The model under review builds one solid part; all positions refer to its coordinate system, in mm. A direction names the side the tool comes from. Give positions to 0.01 mm unless a question says otherwise; leave off trailing zeros. Loops run counter-clockwise (first coordinate to the right, second up) from the corner with the lowest first, then second, coordinate; pieces in that order, holes last. Notation, with made-up numbers: M -16,-7 L 0,-7 A17 cw 0,22 Z; hole C 35,-26.75 d8. An arc over 180 degrees is marked long. One line per item, written item: value. Start each with the question number.
Q1. We need section C-C on y = 0.7. Give the number of separate pieces and of enclosed holes in the cut face, plus the area to 3 significant figures.
Q2. We need section B-B on x = -39. Write out the cut boundary in (y, z).
Q3. For faces 1 (the face through (46.52, 0.69, 39.04)), 2 (the face through (-46.57, 0.69, 38.98)), 3 (the face through (-44.7, 0.69, -45.04)), 4 (the face through (-38.86, 0.689, 46.664)), 5 (the face through (38.86, 0.689, -46.664)), list the 3-axis set-ups (+Z, -Z, +X, -X, +Y, -Y) from which the entire face can be reached by the end or side of a thin tool; tool diameter is ignored.
Q4. Mouldability with a two-part tool opening along Z and no side actions: class faces 6 (the face through (-39.9, 0.7, -25.7)), 7 (the face through (44.7, 0.69, 45.04)), 8 (the face through (-38.8, 0.69, -46.71)), 9 (the face through (-1, 1.397, -1)) as released by +Z, released by -Z, zero draft, split by the parting line, or undercut.
Q5. We need section A-A on z = 24.5. Write out the cut boundary in (x, y), plus the area to 3 significant figures.
Q6. We need section D-D on z = -38. Write out the cut boundary in (x, y), plus the area to 3 significant figures.
Q7. To check wall thickness, follow line 1 along X through (y, z) = (0.5, -36); line 2 along Z through (x, y) = (-40, 1.3); line 3 along X through (y, z) = (0.5, 35). State the ranges of each line that lie inside material, in increasing order. Write a range as from..to.
```python
from build123d import *

# Parameters (mm, degrees)
SKETCH1_R           = 1.016000002
SKETCH1_R_2         = 1.015999994
SKETCH1_R_3         = 1.016000004
SKETCH1_R_4         = 1.016000003
SKETCH1_R_5         = 1.5
BOSS_EXTRUDE1_DEPTH = 1.397


with BuildPart() as part:
    # Sketch1 → Boss-Extrude1 (new body)
    with BuildSketch(Plane(origin=(0, 0, 0), x_dir=(1, 0, 0), z_dir=(0, 1, 0))):
        with BuildLine():
            Line((-44.657487237, -41.209177315), (-46.396043566, -42.947733643))
            ThreePointArc((-46.396043566, -42.947733643), (-46.47043426, -43.125880979), (-46.398093321, -43.304870469))
            Line((-46.398093321, -43.304870469), (-43.050556902, -46.730153436))
            ThreePointArc((-43.050556902, -46.730153436), (-42.865374913, -46.831022486), (-42.667823962, -46.757262364))
            Line((-42.667823962, -46.757262364), (-40.871772737, -44.96121114))
            ThreePointArc((-40.871772737, -44.96121114), (-38.831009329, -46.687575031), (-36.702263747, -48.304204185))
            ThreePointArc((-36.702263747, -48.304204185), (-35.216668272, -49.053976946), (-33.572746514, -49.312190732))
            Line((-33.572746514, -49.312190732), (33.572746514, -49.312190732))
            ThreePointArc((33.572746514, -49.312190732), (35.216668272, -49.053976946), (36.702263747, -48.304204185))
            ThreePointArc((36.702263747, -48.304204185), (38.831009329, -46.687575031), (40.871772737, -44.96121114))
            Line((40.871772737, -44.96121114), (42.667823962, -46.757262364))
            ThreePointArc((42.667823962, -46.757262364), (42.865374913, -46.831022486), (43.050556902, -46.730153436))
            Line((43.050556902, -46.730153436), (46.398093321, -43.304870469))
            ThreePointArc((46.398093321, -43.304870469), (46.47043426, -43.125880979), (46.396043566, -42.947733643))
            Line((46.396043566, -42.947733643), (44.657487237, -41.209177315))
            ThreePointArc((44.657487237, -41.209177315), (46.545191327, -39.007785053), (48.304204175, -36.702263762))
            ThreePointArc((48.304204175, -36.702263762), (49.053976936, -35.216668286), (49.312190722, -33.572746527))
            Line((49.312190722, -33.572746527), (49.312190722, 33.572746527))
            ThreePointArc((49.312190722, 33.572746527), (49.053976936, 35.216668286), (48.304204175, 36.702263762))
            ThreePointArc((48.304204175, 36.702263762), (46.545191327, 39.007785053), (44.657487237, 41.209177315))
            Line((44.657487237, 41.209177315), (46.396043566, 42.947733643))
            ThreePointArc((46.396043566, 42.947733643), (46.47043426, 43.125880979), (46.398093321, 43.304870469))
            Line((46.398093321, 43.304870469), (43.050556902, 46.730153436))
            ThreePointArc((43.050556902, 46.730153436), (42.865374913, 46.831022486), (42.667823962, 46.757262364))
            Line((42.667823962, 46.757262364), (40.871772737, 44.96121114))
            ThreePointArc((40.871772737, 44.96121114), (38.831009329, 46.687575031), (36.702263747, 48.304204185))
            ThreePointArc((36.702263747, 48.304204185), (35.216668272, 49.053976946), (33.572746514, 49.312190732))
            Line((33.572746514, 49.312190732), (-33.572746514, 49.312190732))
            ThreePointArc((-33.572746514, 49.312190732), (-35.216668272, 49.053976946), (-36.702263747, 48.304204185))
            ThreePointArc((-36.702263747, 48.304204185), (-38.831009329, 46.687575031), (-40.871772737, 44.96121114))
            Line((-40.871772737, 44.96121114), (-42.667823962, 46.757262364))
            ThreePointArc((-42.667823962, 46.757262364), (-42.865374913, 46.831022486), (-43.050556902, 46.730153436))
            Line((-43.050556902, 46.730153436), (-46.398093321, 43.304870469))
            ThreePointArc((-46.398093321, 43.304870469), (-46.47043426, 43.125880979), (-46.396043566, 42.947733643))
            Line((-46.396043566, 42.947733643), (-44.657487237, 41.209177315))
            ThreePointArc((-44.657487237, 41.209177315), (-46.545191327, 39.007785053), (-48.304204175, 36.702263762))
            ThreePointArc((-48.304204175, 36.702263762), (-49.053976936, 35.216668286), (-49.312190722, 33.572746527))
            Line((-49.312190722, 33.572746527), (-49.312190722, -33.572746527))
            ThreePointArc((-49.312190722, -33.572746527), (-49.053976936, -35.216668286), (-48.304204175, -36.702263762))
            ThreePointArc((-48.304204175, -36.702263762), (-46.545191327, -39.007785053), (-44.657487237, -41.209177315))
        make_face()
        with Locations(Location((-35.273880312, -43.8949262, 0), (0, 0, 90))):
            Circle(SKETCH1_R, mode=Mode.SUBTRACT)
        with Locations(Location((-43.89492619, -35.273880325, 0), (0, 0, 270))):
            Circle(SKETCH1_R_2, mode=Mode.SUBTRACT)
        with Locations(Location((-31.299173987, -31.299173994, 0), (0, 0, 270))):
            Circle(SKETCH1_R, mode=Mode.SUBTRACT)
        with Locations(Location((43.89492619, -35.273880325, 0), (0, 0, 90))):
            Circle(SKETCH1_R_3, mode=Mode.SUBTRACT)
        with Locations(Location((35.273880312, -43.8949262, 0), (0, 0, 270))):
            Circle(SKETCH1_R_3, mode=Mode.SUBTRACT)
        with Locations(Location((31.299173987, -31.299173994, 0), (0, 0, 90))):
            Circle(SKETCH1_R, mode=Mode.SUBTRACT)
        with Locations(Location((-35.273880312, 43.8949262, 0), (0, 0, 270))):
            Circle(SKETCH1_R, mode=Mode.SUBTRACT)
        with Locations(Location((-31.299173987, 31.299173994, 0), (0, 0, 90))):
            Circle(SKETCH1_R, mode=Mode.SUBTRACT)
        with Locations(Location((-43.89492619, 35.273880325, 0), (0, 0, 90))):
            Circle(SKETCH1_R, mode=Mode.SUBTRACT)
        with Locations(Location((43.89492619, 35.273880325, 0), (0, 0, 270))):
            Circle(SKETCH1_R_4, mode=Mode.SUBTRACT)
        with Locations(Location((35.273880312, 43.8949262, 0), (0, 0, 90))):
            Circle(SKETCH1_R_3, mode=Mode.SUBTRACT)
        with Locations(Location((31.299173987, 31.299173994, 0), (0, 0, 270))):
            Circle(SKETCH1_R, mode=Mode.SUBTRACT)
        with Locations(Location((-39, 24.5, 0), (0, 0, 270))):
            Circle(SKETCH1_R_5, mode=Mode.SUBTRACT)
        with Locations(Location((19, 24.5, 0), (0, 0, 270))):
            Circle(SKETCH1_R_5, mode=Mode.SUBTRACT)
        with Locations(Location((19.002972949, -24.499403884, 0), (0, 0, 270))):
            Circle(SKETCH1_R_5, mode=Mode.SUBTRACT)
        with Locations(Location((-39, -24.5, 0), (0, 0, 270))):
            Circle(SKETCH1_R_5, mode=Mode.SUBTRACT)
    extrude(amount=BOSS_EXTRUDE1_DEPTH)


solid = part.part
```
Solved:
1. separate pieces: 1
1. enclosed holes: 16
1. area: 9,370 mm2
2. outline: M 0,-46.55 L 1.4,-46.55 L 1.4,-26 L 0,-26 Z; M 0,-23 L 1.4,-23 L 1.4,23 L 0,23 Z; M 0,26 L 1.4,26 L 1.4,46.55 L 0,46.55 Z
3. face 1: +X, +Y, -Y
3. face 2: -X, +Y, -Y
3. face 3: -Z, -X, +Y, -Y
3. face 4: +Z, +Y, -Y
3. face 5: -Z, +Y, -Y
4. face 6: undercut
4. face 7: released by +Z
4. face 8: released by -Z
4. face 9: zero draft
5. outline: M -49.31,0 L -40.5,0 L -40.5,1.4 L -49.31,1.4 Z; M -37.5,0 L 17.5,0 L 17.5,1.4 L -37.5,1.4 Z; M 20.5,0 L 49.31,0 L 49.31,1.4 L 20.5,1.4 Z
5. area: 129 mm2
6. outline: M -47.34,0 L 47.34,0 L 47.34,1.4 L -47.34,1.4 Z
6. area: 132 mm2
7. line 1: -48.73..-44.61, -43.18..43.18, 44.61..48.73
7. line 2: -45.72..-25.62, -23.38..23.38, 25.62..45.72
7. line 3: -49.12..-44.87, -42.92..42.92, 44.87..49.12
